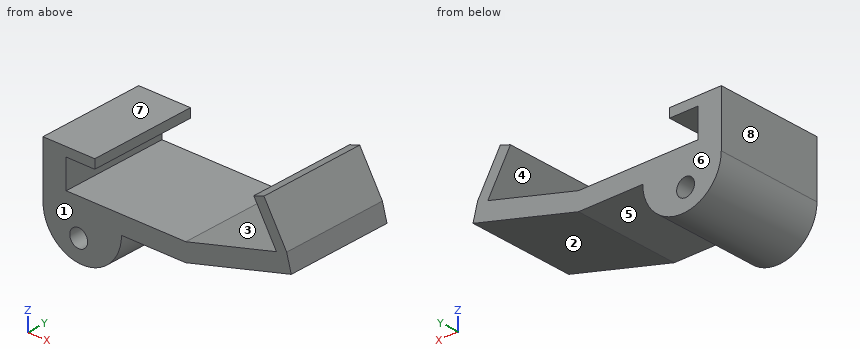
from build123d import *

# Parameters (mm, degrees)
SKETCH1_R           = 0.5
SKETCH1_W           = 1.6
SKETCH1_H           = 0.5
BOSS_EXTRUDE1_DEPTH = 6


with BuildPart() as part:
    # Sketch1 → Boss-Extrude1 (new body)
    with BuildSketch(Plane(origin=(0, 0, 0), x_dir=(1, 0, 0), z_dir=(0, 1, 0))):
        Polygon((4.4, 0), (0, 0), (0, -1), (1.3, -1), (8, -1), (13.081525469, -2.361590646), (13.651326592, -2.549544577), (13.910145637, -1.583618751), (8, 0), align=None)
        Polygon((1.3, -1), (0, -1), (0, -3.1), (1.3, -3.1), (1.3, -2.6), align=None)
        Polygon((12.381156, -4.749544577), (13.651326592, -2.549544577), (13.081525469, -2.361590646), (11.811354877, -4.561590646), align=None)
        with BuildLine():
            ThreePointArc((4.4, 0), (2.2, 2.2), (0, 0))
            Line((0, 0), (4.4, 0))
        make_face()
        with Locations((2, 1)):
            Circle(SKETCH1_R, mode=Mode.SUBTRACT)
        with Locations((2.1, -2.85)):
            Rectangle(SKETCH1_W, SKETCH1_H)
    extrude(amount=BOSS_EXTRUDE1_DEPTH)


solid = part.part
Geometry: final body of the model. Coordinates: model frame, mm. Face numbers are marked on the shaded views. A direction names the side the tool comes from. Give positions to 0.01 mm unless a question says otherwise; leave off trailing zeros. Order: outer loops, then holes, each group sorted by start corner. A loop starts at its lowest first (then second) coordinate and runs counter-clockwise, first axis right, second up. Notation, with made-up numbers: (89.5, -39.5) -> (108.5, -39.5) arc R16 cw to (108.5, -17.5) -> close; hole circle Ø10 at (38.25, 16.5). An arc over 180 degrees is marked (long way). Answer as a JSON object with one key per item and string values.
Q1. Section C-C (x = 2). Output: boundary loops of the cut face in (y, z), plus the area to 3 significant figures.
Entries:
{"outline": "(0, -2.19) -> (6, -2.19) -> (6, -1.5) -> (0, -1.5) -> close; (0, -0.5) -> (6, -0.5) -> (6, 1) -> (0, 1) -> close; (0, 2.6) -> (6, 2.6) -> (6, 3.1) -> (0, 3.1) -> close", "area": "16.1 mm^2"}
Q2. Material intervals for probe 1 along Z at (x, y) = (2, 2.8); probe 2 along X at (y, z) = (1.45, 3); probe 3 along X at (y, z) = (2.35, -1), sorted ascending.
Entries:
{"probe 1": "z = -2.19 to -1.5, -0.5 to 1, 2.6 to 3.1", "probe 2": "x = 0 to 2.9, 12.71 to 13.39", "probe 3": "x = 0.24 to 1.5, 2.5 to 4.16"}
Q3. Draft query along Z for the marked faces 1, 2 and 3. Return one class per face: released by +Z, released by -Z, zero draft, split by the parting line, or undercut.
Entries:
{"face 1": "zero draft", "face 2": "released by -Z", "face 3": "undercut"}
Q4. Section B-B (z = -1). Output: boundary loops of the cut face in (x, y).
Entries:
{"outline": "(0.24, 0) -> (1.5, 0) -> (1.5, 6) -> (0.24, 6) -> close; (2.5, 0) -> (4.16, 0) -> (4.16, 6) -> (2.5, 6) -> close"}
Q5. Section A-A (y = 3). Output: boundary loops of the cut face in (x, z).
Entries:
{"outline": "(0, 0) arc R2.2 ccw to (4.4, 0) -> (8, 0) -> (13.91, 1.58) -> (13.65, 2.55) -> (12.38, 4.75) -> (11.81, 4.56) -> (13.08, 2.36) -> (8, 1) -> (1.3, 1) -> (1.3, 2.6) -> (2.9, 2.6) -> (2.9, 3.1) -> (0, 3.1) -> close; hole circle Ø1 at (2, -1)"}
Q6. Section D-D (z = 1.25). Output: boundary loops of the cut face in (x, y).
Entries:
{"outline": "(0, 0) -> (1.3, 0) -> (1.3, 6) -> (0, 6) -> close; (8.93, 0) -> (12.67, 0) -> (12.67, 6) -> (8.93, 6) -> close"}
Q7. First-contact query: pin 1 (1.5 mm diameter, centred on x = 1.5, y = 3, fed in from +Z); pin 2 (3 mm diameter, centred on x = 7, y = 1.5, fed in from -Z). Flat tips, straight axial feed; report the tip coordinate or a pass-through.
Entries:
{"pin 1": "stops at z = 3.1", "pin 2": "stops at z = 0"}
Q8. Access query for the marked faces 4, 5, 6, 7 and 8. Directions: +Z, -Z, +X, -X, +Y, -Y. A direction counts if a zero-diameter tool reaches every point of the face in a straight line with its end or side. Return the directions, or none.
Entries:
{"face 4": "+Y, -Y", "face 5": "-Z, +X, +Y, -Y", "face 6": "+Z, -Z, +X, -X, +Y", "face 7": "+Z, -X, +Y, -Y", "face 8": "+Z, -Z, -X, +Y, -Y"}
